from build123d import *

# Parameters (mm, degrees)
SKETCH1_R           = 1.5
BOSS_EXTRUDE1_DEPTH = 6


with BuildPart() as part:
    # Sketch1 → Boss-Extrude1 (new body)
    with BuildSketch(Plane(origin=(0, 0, 0), x_dir=(1, 0, 0), z_dir=(0, 1, 0))):
        with BuildLine():
            Line((0, 0), (-80, 0))
            ThreePointArc((-80, 0), (-90, 10), (-80, 20))
            Line((-80, 20), (-65, 20))
            Line((-65, 20), (-65, 28))
            ThreePointArc((-65, 28), (-62, 31), (-59, 28))
            Line((-59, 28), (-59, 20))
            Line((-59, 20), (0, 20))
            ThreePointArc((0, 20), (10, 10), (0, 0))
        make_face()
        with Locations((-80, 10)):
            Circle(SKETCH1_R, mode=Mode.SUBTRACT)
        with Locations((0, 10)):
            Circle(SKETCH1_R, mode=Mode.SUBTRACT)
        with Locations((-30, 10)):
            Circle(SKETCH1_R, mode=Mode.SUBTRACT)
        with Locations((-62, 28)):
            Circle(SKETCH1_R, mode=Mode.SUBTRACT)
    extrude(amount=BOSS_EXTRUDE1_DEPTH)


solid = part.part
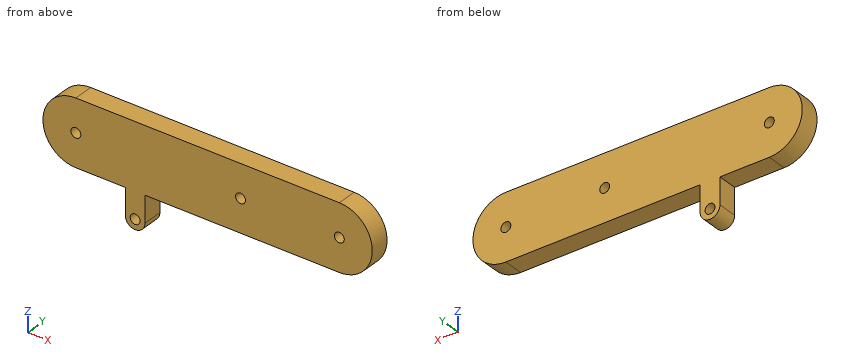
The listing builds one solid part. Answer for the finished solid, in the listing's coordinates (mm). Give positions to 0.01 mm unless a question says otherwise; leave off trailing zeros. Write each loop counter-clockwise with the first axis right and the second up, starting at its lowest first coordinate (ties: lowest second). Pieces come first, ordered by that corner, then holes. Notation, with made-up numbers: (7, 12) -> (51, 12) arc R18 ccw to (51, 23) -> close; hole circle Ø2 at (5.5, 54.25). An arc over 180 degrees is marked (long way). One line per question, with ' | ' between items. Start each with the question number.
1. Section A-A (x = -30) is taken. Determine the outline of the cut face in (y, z), plus the area to 3 significant figures.
2. Given pin 1 Ø8 at (x, z) = (-3.5, -25) entering from -Y; pin 2 Ø1 at (y, z) = (4, -4.5) entering from -X; pin 3 Ø1.8 at (x, y) = (-39.5, 3) entering from -Z; pin 4 Ø1.8 at (y, z) = (2, -23.5) entering from -X, each flat-ended and moving along its own axis, determine where each tip first touches the part or whether it passes through.
3. Section C-C (x = -62) is taken. Determine the outline of the cut face in (y, z), plus the area to 3 significant figures.
4. Find the intervals of material crossed by probe 1 along X at (y, z) = (3.4, -10); probe 2 along Z at (x, y) = (-62, 4.85); probe 3 along X at (y, z) = (3.4, -28), in increasing order.
5. Section B-B (y = 1.9) is taken. Determine the outline of the cut face in (x, z), plus the area to 3 significant figures.
6. Section D-D (z = -4.5) is taken. Determine the outline of the cut face in (x, y).
Response values:
1) outline: (0, -20) -> (6, -20) -> (6, -11.5) -> (0, -11.5) -> close; (0, -8.5) -> (6, -8.5) -> (6, 0) -> (0, 0) -> close | area: 102 mm2
2) pin 1: through | pin 2: x = -88.66 | pin 3: z = -20 | pin 4: x = -65
3) outline: (0, -31) -> (6, -31) -> (6, -29.5) -> (0, -29.5) -> close; (0, -26.5) -> (6, -26.5) -> (6, 0) -> (0, 0) -> close | area: 168 mm2
4) probe 1: -90 to -81.5, -78.5 to -31.5, -28.5 to -1.5, 1.5 to 10 | probe 2: -31 to -29.5, -26.5 to 0 | probe 3: -65 to -63.5, -60.5 to -59
5) outline: (-80, -20) -> (-65, -20) -> (-65, -28) arc R3 ccw to (-59, -28) -> (-59, -20) -> (0, -20) arc R10 ccw to (0, 0) -> (-80, 0) arc R10 ccw to start; hole circle Ø3 at (-80, -10); hole circle Ø3 at (-62, -28); hole circle Ø3 at (-30, -10); hole circle Ø3 at (0, -10) | area: 1,950 mm2
6) outline: (-88.35, 0) -> (8.35, 0) -> (8.35, 6) -> (-88.35, 6) -> close
